Input: part model. Units: mm. Frame: model coordinates. Face numbers are marked on the shaded views. A direction names the side the tool comes from. Round coordinates to 2 decimals unless told otherwise and drop trailing zeros. Order: outer loops, then holes, each group sorted by start corner. A loop starts at its lowest first (then second) coordinate and runs counter-clockwise, first axis right, second up. Notation, with made-up numbers: (-35, 56) -> (14, 56) arc R7 cw to (14, 69) -> close; hole circle Ø9 at (75, 3). An arc over 180 degrees is marked (long way). Use a Markdown table: item, result.
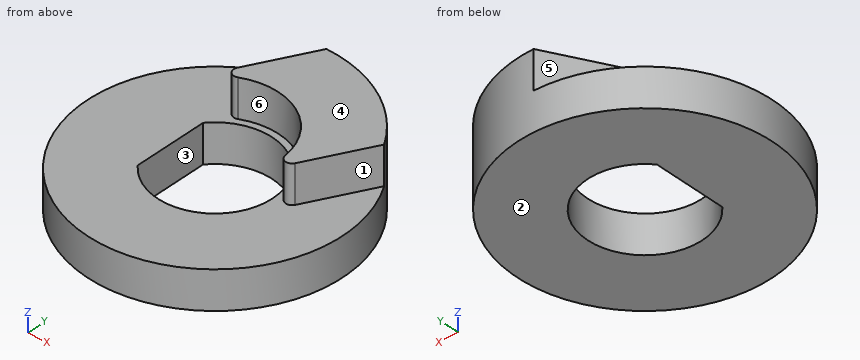
from build123d import *

# Parameters (mm, degrees)
F1_DEPTH = 3
F2_DEPTH = 6
F3_R     = 0.49999


# Not quite as in the source:
# - a fillet or chamfer is up to 0.001 mm smaller than in the source, because OpenCascade refuses the exact size


with BuildPart() as f1:
    # F0 (on Top) → F1 (new body)
    with BuildSketch(Plane.XY):
        with BuildLine():
            ThreePointArc((-0.3210767755, 9.9948441561), (-6.9566239026, -7.1836887375), (10, 0))
            ThreePointArc((10, 0), (9.616457393, 2.7429449883), (8.4952505583, 5.2754827222))
            Line((8.4952505583, 5.2754827222), (4.4081636669, -2.359680717))
            ThreePointArc((4.4081636669, -2.359680717), (2.359680717, 4.4081636669), (-4.4081636669, 2.359680717))
            Line((-4.4081636669, 2.359680717), (-0.3210767755, 9.9948441561))
        make_face()
        with BuildLine():
            ThreePointArc((-3.5, 2.8284271247), (4.5, 0), (-3.5, -2.8284271247))
            Line((-3.5, -2.8284271247), (-3.5, 2.8284271247))
        make_face(mode=Mode.SUBTRACT)
        with BuildLine():
            Line((4.4081636669, -2.359680717), (8.4952505583, 5.2754827222))
            ThreePointArc((8.4952505583, 5.2754827222), (4.7193614339, 8.8163273338), (-0.3210767755, 9.9948441561))
            Line((-0.3210767755, 9.9948441561), (-4.4081636669, 2.359680717))
            ThreePointArc((-4.4081636669, 2.359680717), (2.359680717, 4.4081636669), (4.4081636669, -2.359680717))
        make_face()
    extrude(amount=F1_DEPTH)

    # F0 (on Top) → F2 (join)
    with BuildSketch(Plane.XY):
        with BuildLine():
            Line((4.4081636669, -2.359680717), (8.4952505583, 5.2754827222))
            ThreePointArc((8.4952505583, 5.2754827222), (4.7193614339, 8.8163273338), (-0.3210767755, 9.9948441561))
            Line((-0.3210767755, 9.9948441561), (-4.4081636669, 2.359680717))
            ThreePointArc((-4.4081636669, 2.359680717), (2.359680717, 4.4081636669), (4.4081636669, -2.359680717))
        make_face()
    extrude(amount=F2_DEPTH)

    # F3 (radius 0.5 in the source; OpenCascade refuses exactly that, so slightly less here)
    f3_edges = [f1.edges().sort_by_distance(p)[0] for p in [
        (-4.408164, 2.359681, 4.5),
        (4.408164, -2.359681, 4.5),
    ]]
    fillet(f3_edges, radius=F3_R)


solid = f1.part
1) Cut plane A-A on x = 0. Return loops of the section in (y, z).
Results found:
| item | result |
|---|---|
| outline | (-10, 0) -> (-4.5, 0) -> (-4.5, 3) -> (-10, 3) -> close; (4.5, 0) -> (10, 0) -> (10, 6) -> (5, 6) -> (5, 3) -> (4.5, 3) -> close |
2) Pin query (flat end, axial travel): pin 1 Ø5 at (x, y) = (-6, 6) entering from -Z; pin 2 Ø3 at (y, z) = (2.5, 2.5) entering from +X; pin 3 Ø10 at (x, y) = (4, -5) entering from +Z. Return the tip coordinate at first contact, or that it passes through.
Results found:
| item | result |
|---|---|
| pin 1 | stops at z = 0 |
| pin 2 | stops at x = 9.95 |
| pin 3 | stops at z = 3 |
3) Cut plane B-B on y = -1.75. Return loops of the section in (x, z), and give its area (3 significant figures).
Results found:
| item | result |
|---|---|
| outline | (-9.85, 0) -> (-3.5, 0) -> (-3.5, 3) -> (-9.85, 3) -> close; (4.15, 0) -> (9.85, 0) -> (9.85, 3) -> (4.15, 3) -> close |
| area | 36.1 mm² |
4) Cut plane D-D on y = -4. Return loops of the section in (x, z).
Results found:
| item | result |
|---|---|
| outline | (-9.17, 0) -> (-2.06, 0) -> (-2.06, 3) -> (-9.17, 3) -> close; (2.06, 0) -> (9.17, 0) -> (9.17, 3) -> (2.06, 3) -> close |
5) Cut plane C-C on z = 1. Return loops of the section in (x, y).
Results found:
| item | result |
|---|---|
| outline | circle Ø20 at (0, 0); hole (-3.5, -2.83) arc R4.5 ccw (long way) to (-3.5, 2.83) -> close |
6) Pull-direction query (Y, two-part tool) for the marked faces 3, 4, 5 and 6; classes: +Y half, -Y half, draft (parallel to the pull), parting line (faces both ways), or undercut.
Results found:
| item | result |
|---|---|
| face 3 | undercut |
| face 4 | draft |
| face 5 | +Y half |
| face 6 | -Y half |
7) Set-up query: the marked faces 1 and 2. Return all of +Z, -Z, +X, -X, +Y, -Y with unobstructed straight access to the full face (end or side cutting, diameter ignored); none if empty.
Results found:
| item | result |
|---|---|
| face 1 | +Z, +X, -Y |
| face 2 | -Z, +X, -X, +Y, -Y |
8) Line query: L1, parallel to X at y = 0, z = 1; L2, parallel to Y at x = 0, z = 1.55; L3, parallel to Z at x = 5.25, y = -2.5. Output: solid intervals per line, ascending. Write a range as [from, to].
Results found:
| item | result |
|---|---|
| L1 | x = [-10, -3.5], [4.5, 10] |
| L2 | y = [-10, -4.5], [4.5, 10] |
| L3 | z = [0, 3] |
